from build123d import *

# Parameters (mm, degrees)
SKETCH1_R           = 1.6
BOSS_EXTRUDE1_DEPTH = 5
SKETCH2_W           = 3.6
SKETCH2_H           = 1.5
CUT_EXTRUDE1_DEPTH  = 32.830802692


with BuildPart() as part:
    # Sketch1 → Boss-Extrude1 (new body)
    with BuildSketch(Plane(origin=(0, 0, 0), x_dir=(1, 0, 0), z_dir=(0, 1, 0))):
        with BuildLine():
            Line((-27, 3.6), (0, 3.6))
            ThreePointArc((0, 3.6), (3.6, 0), (0, -3.6))
            Line((0, -3.6), (-27, -3.6))
            ThreePointArc((-27, -3.6), (-30.6, 0), (-27, 3.6))
        make_face()
        with Locations(Location((0, 0, 0), (0, 0, 270))):
            Circle(SKETCH1_R, mode=Mode.SUBTRACT)
        with Locations(Location((-27, 0, 0), (0, 0, 270))):
            Circle(SKETCH1_R, mode=Mode.SUBTRACT)
    extrude(amount=BOSS_EXTRUDE1_DEPTH)

    # Sketch2 → Cut-Extrude1 (cut, through all)
    with BuildSketch(Plane.XY.offset(3.6)):
        Polygon((-16.049747468, 1.5), (-27, 1.5), (-27, 0), (-14.549747468, 0), align=None)
        with Locations((-28.8, 0.75)):
            Rectangle(SKETCH2_W, SKETCH2_H)
        Polygon((0, 5), (-14.6, 5), (-13.1, 3.5), (0, 3.5), align=None)
        with Locations((1.8, 4.25)):
            Rectangle(SKETCH2_W, SKETCH2_H)
    extrude(amount=-CUT_EXTRUDE1_DEPTH, mode=Mode.SUBTRACT)


solid = part.part
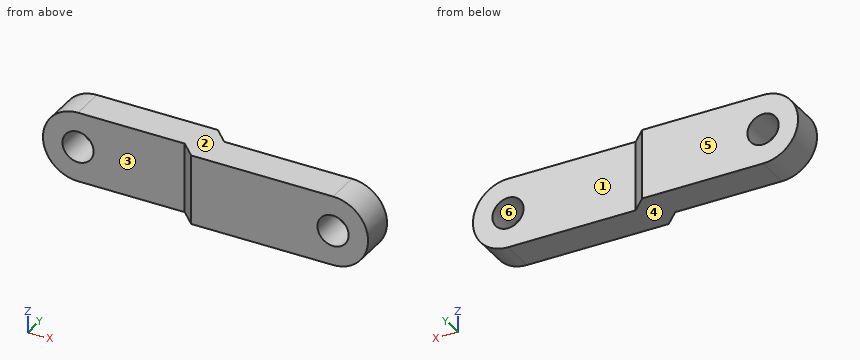
Design review of the part built by this model. Coordinates are the model's own, in mm. Face numbers are marked on the shaded views. A direction names the side the tool comes from. Coordinates: 2 decimals unless noted, no trailing zeros. Loops run counter-clockwise (first coordinate to the right, second up) from the corner with the lowest first, then second, coordinate; pieces in that order, holes last.
Item 1: Wall thickness on L1, parallel to X at y = 2.8, z = 0; L2, parallel to Z at x = 0, y = 1.2; L3, parallel to X at y = 3.25, z = -1: over which ranges is each line inside the solid? List them lowest first.
Completed:
L1: x = -30.6 to -28.6, -25.4 to -1.6, 1.6 to 3.6
L2: z = -3.6 to -1.6, 1.6 to 3.6
L3: x = -30.46 to -28.25, -25.75 to -1.25, 1.25 to 3.46
Item 2: Add section D-D (x = -21.5). Write out the cut boundary in (y, z), and give its area (3 significant figures).
Completed:
outline: (1.5, -3.6) - (5, -3.6) - (5, 3.6) - (1.5, 3.6) - close
area: 25.2 mm2
Item 3: Clearance check with flat-ended pins moving along their axes: pin 1 (2 mm diameter, centred on x = -1, z = 0, fed in from +Y); pin 2 (3 mm diameter, centred on x = 0, z = 0, fed in from -Y). State where each tip first meets the part, or that it passes through.
Completed:
pin 1: stops at y = 3.5
pin 2: passes through
Item 4: Add section C-C (y = 3.15). Write out the cut boundary in (x, z), and give its area (3 significant figures).
Completed:
outline: (-27, -3.6) - (0, -3.6) arc R3.6 ccw to (0, 3.6) - (-27, 3.6) arc R3.6 ccw to start; hole circle Ø3.2 at (-27, 0); hole circle Ø3.2 at (0, 0)
area: 219 mm2
Item 5: For the marked faces 1, 2 and 3, list the 3-axis set-ups (+Z, -Z, +X, -X, +Y, -Y) from which the entire face can be reached by the end or side of a thin tool; tool diameter is ignored.
Completed:
face 1: +Z, -Z, +X, +Y
face 2: +Z, +X, -X, +Y, -Y
face 3: +Z, -Z, -X, -Y
Item 6: Add section B-B (y = 4.4). Write out the cut boundary in (x, z), and give its area (3 significant figures).
Completed:
outline: (-27, -3.6) - (-14, -3.6) - (-14, 3.6) - (-27, 3.6) arc R3.6 ccw to start; hole circle Ø3.2 at (-27, 0)
area: 106 mm2
Item 7: Draft analysis for pull direction Z (two halves, no side actions). For the marked faces 4, 5 and 6, state which applies: pulls with the +Z half, pulls with the -Z half, needs draft (parallel to the pull), parting line crosses it, or undercut.
Completed:
face 4: pulls with the -Z half
face 5: needs draft
face 6: undercut
Item 8: Add section A-A (z = 0). Write out the cut boundary in (x, y).
Completed:
outline: (-30.6, 1.5) - (-28.6, 1.5) - (-28.6, 5) - (-30.6, 5) - close; (-25.4, 1.5) - (-16.05, 1.5) - (-14.55, 0) - (-1.6, 0) - (-1.6, 3.5) - (-13.1, 3.5) - (-14.6, 5) - (-25.4, 5) - close; (1.6, 0) - (3.6, 0) - (3.6, 3.5) - (1.6, 3.5) - close
